```python
from build123d import *

# Parameters (mm, degrees)
SM_BASE_FLANGE_1_DEPTH = 2066
CUT_EXTRUDE_2_DEPTH    = 2.3
CUT_EXTRUDE_3_REACH    = 2082.367
CUT_EXTRUDE_4_REACH    = 2086.839
SKETCH_8_R             = 7


# Sheet-metal steps are written as plain solids
with BuildPart() as part:
    # Sketch 1 → Sm Base Flange 1 (new body)
    with BuildSketch(Plane.XY):
        with BuildLine():
            Line((-35, 15), (-35, 1))
            ThreePointArc((-35, 1), (-34.707106781, 0.292893219), (-34, 0))
            Line((-34, 0), (-1, 0))
            ThreePointArc((-1, 0), (-0.292893219, 0.292893219), (0, 1))
            Line((0, 1), (0, 49.7))
            ThreePointArc((0, 49.7), (0.966547622, 52.033452378), (3.3, 53))
            Line((3.3, 53), (22.085786438, 53))
            ThreePointArc((22.085786438, 53), (22.46846987, 53.076120467), (22.792893219, 53.292893219))
            Line((22.792893219, 53.292893219), (32.166547622, 62.666547622))
            ThreePointArc((32.166547622, 62.666547622), (34.5, 63.633095244), (36.833452378, 62.666547622))
            Line((36.833452378, 62.666547622), (46.207106781, 53.292893219))
            ThreePointArc((46.207106781, 53.292893219), (46.53153013, 53.076120467), (46.914213562, 53))
            Line((46.914213562, 53), (102.085786438, 53))
            ThreePointArc((102.085786438, 53), (102.46846987, 53.076120467), (102.792893219, 53.292893219))
            Line((102.792893219, 53.292893219), (112.166547622, 62.666547622))
            ThreePointArc((112.166547622, 62.666547622), (114.5, 63.633095244), (116.833452378, 62.666547622))
            Line((116.833452378, 62.666547622), (126.207106781, 53.292893219))
            ThreePointArc((126.207106781, 53.292893219), (126.53153013, 53.076120467), (126.914213562, 53))
            Line((126.914213562, 53), (182.085786438, 53))
            ThreePointArc((182.085786438, 53), (182.46846987, 53.076120467), (182.792893219, 53.292893219))
            Line((182.792893219, 53.292893219), (192.166547622, 62.666547622))
            ThreePointArc((192.166547622, 62.666547622), (194.5, 63.633095244), (196.833452378, 62.666547622))
            Line((196.833452378, 62.666547622), (206.207106781, 53.292893219))
            ThreePointArc((206.207106781, 53.292893219), (206.53153013, 53.076120467), (206.914213562, 53))
            Line((206.914213562, 53), (231.7, 53))
            ThreePointArc((231.7, 53), (234.033452378, 52.033452378), (235, 49.7))
            Line((235, 49.7), (235, 3.3))
            ThreePointArc((235, 3.3), (234.033452378, 0.966547622), (231.7, 0))
            Line((231.7, 0), (202, 0))
            Line((202, 0), (202, 2.3))
            Line((202, 2.3), (231.7, 2.3))
            ThreePointArc((231.7, 2.3), (232.407106781, 2.592893219), (232.7, 3.3))
            Line((232.7, 3.3), (232.7, 49.7))
            ThreePointArc((232.7, 49.7), (232.407106781, 50.407106781), (231.7, 50.7))
            Line((231.7, 50.7), (206.914213562, 50.7))
            ThreePointArc((206.914213562, 50.7), (205.651358236, 50.951197543), (204.580761184, 51.666547622))
            Line((204.580761184, 51.666547622), (195.207106781, 61.040202025))
            ThreePointArc((195.207106781, 61.040202025), (194.5, 61.333095244), (193.792893219, 61.040202025))
            Line((193.792893219, 61.040202025), (184.419238816, 51.666547622))
            ThreePointArc((184.419238816, 51.666547622), (183.348641764, 50.951197543), (182.085786438, 50.7))
            Line((182.085786438, 50.7), (126.914213562, 50.7))
            ThreePointArc((126.914213562, 50.7), (125.651358236, 50.951197543), (124.580761184, 51.666547622))
            Line((124.580761184, 51.666547622), (115.207106781, 61.040202025))
            ThreePointArc((115.207106781, 61.040202025), (114.5, 61.333095244), (113.792893219, 61.040202025))
            Line((113.792893219, 61.040202025), (104.419238816, 51.666547622))
            ThreePointArc((104.419238816, 51.666547622), (103.348641764, 50.951197543), (102.085786438, 50.7))
            Line((102.085786438, 50.7), (46.914213562, 50.7))
            ThreePointArc((46.914213562, 50.7), (45.651358236, 50.951197543), (44.580761184, 51.666547622))
            Line((44.580761184, 51.666547622), (35.207106781, 61.040202025))
            ThreePointArc((35.207106781, 61.040202025), (34.5, 61.333095244), (33.792893219, 61.040202025))
            Line((33.792893219, 61.040202025), (24.419238816, 51.666547622))
            ThreePointArc((24.419238816, 51.666547622), (23.348641764, 50.951197543), (22.085786438, 50.7))
            Line((22.085786438, 50.7), (3.3, 50.7))
            ThreePointArc((3.3, 50.7), (2.592893219, 50.407106781), (2.3, 49.7))
            Line((2.3, 49.7), (2.3, 1))
            ThreePointArc((2.3, 1), (1.333452378, -1.333452378), (-1, -2.3))
            Line((-1, -2.3), (-34, -2.3))
            ThreePointArc((-34, -2.3), (-36.333452378, -1.333452378), (-37.3, 1))
            Line((-37.3, 1), (-37.3, 15))
            Line((-37.3, 15), (-35, 15))
        make_face()
    extrude(amount=SM_BASE_FLANGE_1_DEPTH)

    # Sketch 6 → Cut-Extrude 2 (cut)
    with BuildSketch(Plane.XZ):
        with BuildLine():
            Line((213.5, 2055.5), (213.5, 2045.5))
            ThreePointArc((213.5, 2045.5), (219, 2040), (224.5, 2045.5))
            Line((224.5, 2045.5), (224.5, 2055.5))
            ThreePointArc((224.5, 2055.5), (219, 2061), (213.5, 2055.5))
        make_face()
    cut_extrude_2 = extrude(amount=-CUT_EXTRUDE_2_DEPTH, mode=Mode.SUBTRACT)

    # Sketch 7 → Cut-Extrude 3 (cut, up to next)
    with BuildSketch(Plane.XZ.offset(2.3), mode=Mode.PRIVATE) as cut_extrude_3_sk1:
        with BuildLine():
            Line((-10.5, 2045.5), (-10.5, 2055.5))
            ThreePointArc((-10.5, 2055.5), (-16, 2061), (-21.5, 2055.5))
            Line((-21.5, 2055.5), (-21.5, 2045.5))
            ThreePointArc((-21.5, 2045.5), (-16, 2040), (-10.5, 2045.5))
        make_face()
    cut_extrude_3_tool1 = extrude(cut_extrude_3_sk1.sketch, amount=-CUT_EXTRUDE_3_REACH, mode=Mode.PRIVATE) & part.part
    cut_extrude_3 = cut_extrude_3_tool1.solids().sort_by_distance((-16, -2.3, 2050.5))[0]
    add(cut_extrude_3, mode=Mode.SUBTRACT)

    # Mirror 1: Cut-Extrude 2, Cut-Extrude 3 across plane
    add(cut_extrude_2.mirror(Plane.XY.offset(1033)), mode=Mode.SUBTRACT)
    add(cut_extrude_3.mirror(Plane.XY.offset(1033)), mode=Mode.SUBTRACT)

    # Cut-Extrude 4: up to this face of the body (flat: up to its plane)
    cut_extrude_4_end = Plane(part.part.faces().sort_by_distance((0, 25.35, 1033))[0])
    # Sketch 8 → Cut-Extrude 4 (cut, up to the picked face)
    with BuildSketch(Plane(origin=(235, 0, 0), x_dir=(0, 0, -1), z_dir=(1, 0, 0)), mode=Mode.PRIVATE) as cut_extrude_4_sk1:
        with Locations((-2036, 28)):
            Circle(SKETCH_8_R)
    cut_extrude_4_tool1 = split(extrude(cut_extrude_4_sk1.sketch, amount=-CUT_EXTRUDE_4_REACH, mode=Mode.PRIVATE), bisect_by=cut_extrude_4_end, keep=Keep.BOTH, mode=Mode.PRIVATE)
    # Sketch 8 → Cut-Extrude 4 (cut, up to the picked face)
    with BuildSketch(Plane(origin=(235, 0, 0), x_dir=(0, 0, -1), z_dir=(1, 0, 0)), mode=Mode.PRIVATE) as cut_extrude_4_sk2:
        with Locations((-1986, 28)):
            Circle(SKETCH_8_R)
    cut_extrude_4_tool2 = split(extrude(cut_extrude_4_sk2.sketch, amount=-CUT_EXTRUDE_4_REACH, mode=Mode.PRIVATE), bisect_by=cut_extrude_4_end, keep=Keep.BOTH, mode=Mode.PRIVATE)
    # Sketch 8 → Cut-Extrude 4 (cut, up to the picked face)
    with BuildSketch(Plane(origin=(235, 0, 0), x_dir=(0, 0, -1), z_dir=(1, 0, 0)), mode=Mode.PRIVATE) as cut_extrude_4_sk3:
        with Locations((-1936, 28)):
            Circle(SKETCH_8_R)
    cut_extrude_4_tool3 = split(extrude(cut_extrude_4_sk3.sketch, amount=-CUT_EXTRUDE_4_REACH, mode=Mode.PRIVATE), bisect_by=cut_extrude_4_end, keep=Keep.BOTH, mode=Mode.PRIVATE)
    cut_extrude_4_1 = cut_extrude_4_tool1.solids().sort_by(Axis((235, 28, 2036), (-1, 0, 0)))[0]
    add(cut_extrude_4_1, mode=Mode.SUBTRACT)
    cut_extrude_4_2 = cut_extrude_4_tool2.solids().sort_by(Axis((235, 28, 1986), (-1, 0, 0)))[0]
    add(cut_extrude_4_2, mode=Mode.SUBTRACT)
    cut_extrude_4_3 = cut_extrude_4_tool3.solids().sort_by(Axis((235, 28, 1936), (-1, 0, 0)))[0]
    add(cut_extrude_4_3, mode=Mode.SUBTRACT)
    cut_extrude_4 = cut_extrude_4_1 + cut_extrude_4_2 + cut_extrude_4_3  # Cut-Extrude 4 as one shape, for the pattern or mirror that repeats it

    # Mirror 2: Cut-Extrude 4 across plane
    add(cut_extrude_4.mirror(Plane.XY.offset(1033)), mode=Mode.SUBTRACT)


solid = part.part
```
Geometry: final body of the model. Coordinates: model frame, mm. A direction names the side the tool comes from. Coordinates: 2 decimals unless noted, no trailing zeros. Write each question's results on one line, items separated by ' | '.
1) Line query: line 1 (X direction, y = 6.5, z = 532); line 2 (X direction, y = 38, z = 1230.5); line 3 (X direction, y = 58, z = 1338.5). Output: solid intervals per line, ascending. Write a range as from..to.
Results list:
line 1: -37.3..-35, 0..2.3, 232.7..235 | line 2: 0..2.3, 232.7..235 | line 3: 27.5..30.75, 38.25..41.5, 107.5..110.75, 118.25..121.5, 187.5..190.75, 198.25..201.5
2) Pull-direction query (Y, two-part tool) for faces 1 (the flat face through (154, 53, 1019)), 2 (the flat face through (155, 50.7, 1019)), 3 (the flat face through (235, 27, 1019)), 4 (the flat face through (232.7, 26, 1019)); classes: pulls with the +Y half, pulls with the -Y half, needs draft (parallel to the pull), parting line crosses it, or undercut.
Results list:
face 1: pulls with the +Y half | face 2: pulls with the -Y half | face 3: needs draft | face 4: undercut
3) Set-up query: faces 5 (the flat face through (0, 25, 1019)), 6 (the flat face through (110, 58, 2066)), 7 (the flat face through (2.3, 26, 1019)). Return all of +Z, -Z, +X, -X, +Y, -Y with unobstructed straight access to the full face (end or side cutting, diameter ignored); none if empty.
Results list:
face 5: +Z, -Z, +Y | face 6: +Z, +X, -X, +Y, -Y | face 7: +Z, -Z, -Y
4) Pin query (flat end, axial travel): pin 1 (4 mm diameter, centred on y = 19, z = 675.5, fed in from -X); pin 2 (0.7 mm diameter, centred on y = -1.5, z = 2050, fed in from -X); pin 3 (15 mm diameter, centred on x = 15.5, z = 1131.5, fed in from +Y); pin 4 (5 mm diameter, centred on x = 171.5, y = 47, fed in from -Z). Return the tip coordinate at first contact, or that it passes through.
Results list:
pin 1: x = 0 | pin 2: x = -36.5 | pin 3: y = 53.5 | pin 4: through
